```python
from build123d import *

# Parameters (mm, degrees)
F1_DEPTH = 603.25
F3_DEPTH = 38.101


with BuildPart() as f1:
    # F0 (on Front) → F1 (new body, symmetric)
    with BuildSketch(Plane.XZ):
        Polygon((-19.05, -31.75), (19.05, -31.75), (19.05, 31.75), (11.1125, 31.75), (11.1125, 21.59), (7.9375, 21.59), (7.9375, 31.75), (-7.9375, 31.75), (-7.9375, 21.59), (-11.1125, 21.59), (-11.1125, 31.75), (-19.05, 31.75), align=None)
    extrude(amount=F1_DEPTH, both=True)

    # F2 (on face) → F3 (cut, through all)
    with BuildSketch(Plane(origin=(-19.05, 0, 0), x_dir=(0, -1, 0), z_dir=(-1, 0, 0))):
        Polygon((539.75, 31.75), (603.25, -31.75), (603.25, 31.75), align=None)
        Polygon((-603.25, 31.75), (-603.25, -31.75), (-539.75, 31.75), align=None)
    extrude(amount=-F3_DEPTH, mode=Mode.SUBTRACT)


solid = f1.part
```
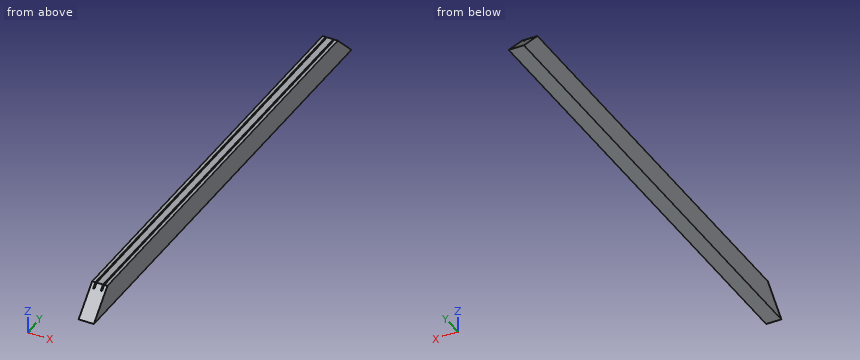
Verification items for the finished model (mm, model axes). Coordinates: 2 decimals unless noted, no trailing zeros. Order: outer loops, then holes, each group sorted by start corner. A loop starts at its lowest first (then second) coordinate and runs counter-clockwise, first axis right, second up. Notation, with made-up numbers: (-24, -31) - (8, -31) arc R17 cw to (8, -11) - close; hole circle Ø9 at (2, 87). An arc over 180 degrees is marked (long way). Return JSON: item names as keys, results as strings.
(1) Section check A-A, the plane y = -133. Record the cut outline in (x, z), and give its area (3 significant figures).
Filled sheet:
{"outline": "(-19.05, -31.75) - (19.05, -31.75) - (19.05, 31.75) - (11.11, 31.75) - (11.11, 21.59) - (7.94, 21.59) - (7.94, 31.75) - (-7.94, 31.75) - (-7.94, 21.59) - (-11.11, 21.59) - (-11.11, 31.75) - (-19.05, 31.75) - close", "area": "2,350 mm^2"}
(2) Section check B-B, the plane z = -10.5. Record the cut outline in (x, y).
Filled sheet:
{"outline": "(-19.05, -582) - (19.05, -582) - (19.05, 582) - (-19.05, 582) - close"}
(3) Thickness scan on line 1 along X through (y, z) = (540.5, 29); line 2 along Z through (x, y) = (8, -382); line 3 along Y through (x, z) = (15, 28). Record the ranges inside material, lowest first.
Filled sheet:
{"line 1": "x = -19.05 to -11.11, -7.94 to 7.94, 11.11 to 19.05", "line 2": "z = -31.75 to 21.59", "line 3": "y = -543.5 to 543.5"}
(4) Section check C-C, the plane x = 0. Record the cut outline in (y, z), and give its area (3 significant figures).
Filled sheet:
{"outline": "(-603.25, -31.75) - (603.25, -31.75) - (539.75, 31.75) - (-539.75, 31.75) - close", "area": "72,600 mm^2"}
(5) Go/stop test with flat-tipped pins: pin 1 (2 mm diameter, centred on x = -12, z = -24, fed in from +Y); pin 2 (3 mm diameter, centred on x = -11, z = -6, fed in from -Y); pin 3 (4 mm diameter, centred on x = -13.5, z = 20.5, fed in from -Y). Record where each tip stops, or that it passes through.
Filled sheet:
{"pin 1": "stops at y = 596.5", "pin 2": "stops at y = -579", "pin 3": "stops at y = -553"}
